CAD build for the part. Positions are in the model's coordinates, mm. Give positions to 0.01 mm unless a question says otherwise; leave off trailing zeros. Loops run counter-clockwise (first coordinate to the right, second up) from the corner with the lowest first, then second, coordinate; pieces in that order, holes last. Notation, with made-up numbers: (60, -22) -> (70, -22) arc R14 cw to (70, -15) -> close; hole circle Ø5 at (73.5, -21). An arc over 180 degrees is marked (long way). Use one line per item in the form item = value.
Autodesk Fusion 360 part; units mm, degrees
sketch "Sketch1" plane through (0, 0, 0) normal (0, 1, 0) x (1, 0, 0)
  line L0 (0, 0) -> (31.94, 0)
  line L1 (31.94, 0) -> (31.94, 1.3)
  line L2 (31.94, 1.3) -> (0, 1.3)
  line L3 (0, 1.3) -> (0, 0)
  dimension "d13" = 1.3
extrude "Extrude1" add sketch "Sketch1" along normal blind 55
sketch "Sketch3" plane through (0, 0, 0) normal (0, -1, 0) x (1, 0, 0)
  line L0 (0, 0) -> (0, -1.3)
  line L1 (0, -1.3) -> (31.94, -1.3)
  line L2 (31.94, -1.3) -> (31.94, 0)
  line L3 (31.94, 0) -> (0, 0)
  line L4 (5.44, 0) -> (26.5, 0)
  line L5 (26.5, 0) -> (26.5, 3)
  line L6 (26.5, 3) -> (5.44, 3)
  line L7 (5.44, 3) -> (5.44, 0)
extrude "Extrude2" add sketch "Sketch3" against normal blind 1 contours L3 L4 L5 L6 L7
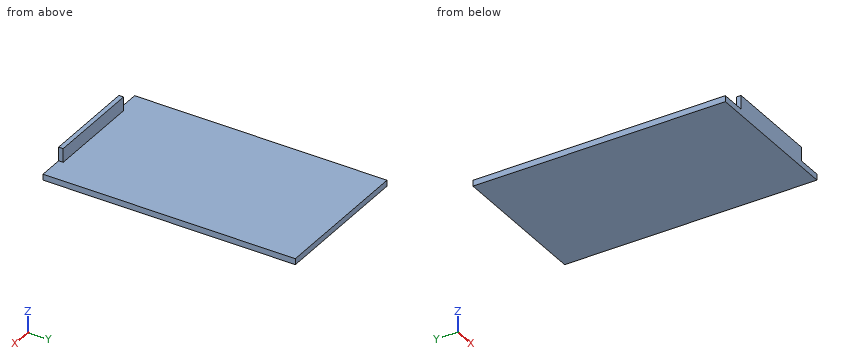
1. Cut at C-C, the plane z = 1.2. Write the cut outline in (x, y), then the cut area to 3 significant figures.
Result sheet:
outline = (5.44, 0) -> (26.5, 0) -> (26.5, 1) -> (5.44, 1) -> close
area = 21.1 mm^2
2. Cut at A-A, the plane y = 23. Write the cut outline in (x, z), then the cut area to 3 significant figures.
Result sheet:
outline = (0, -1.3) -> (31.94, -1.3) -> (31.94, 0) -> (0, 0) -> close
area = 41.5 mm^2
3. Cut at B-B, the plane x = 14.5. Write the cut outline in (y, z).
Result sheet:
outline = (0, -1.3) -> (55, -1.3) -> (55, 0) -> (1, 0) -> (1, 3) -> (0, 3) -> close
4. Drop flat-ended pins along their axis: P1, Ø1, axis at x = 11, y = 44, coming from the +Z side; P2, Ø1.5, axis at x = 16, z = 1, coming from the +Y side; P3, Ø1.1, axis at y = 0.5, z = 1, coming from the -X side. Give the stop position or say it passes through.
Result sheet:
P1 = 0
P2 = 1
P3 = 5.44
5. Drill centre lines: line 1 (Z direction, x = 5.5, y = 46); line 2 (Y direction, x = 22.5, z = 2.55). Where is each one in solid material? Low to high.
Result sheet:
line_1 = -1.3 to 0
line_2 = 0 to 1
